```python
from build123d import *

# Parameters (mm, degrees)
F0_W          = 571.5
F0_H          = 19.05
F1_DEPTH      = 88.9
F2_W          = 88.9
F2_H          = 19.05
F3_DEPTH      = 6.35
F4_W          = 88.9
F4_H          = 19.05
F5_DEPTH      = 6.35
F5_DEPTH_BACK = 25.4


with BuildPart() as f1:
    # F0 (on Front) → F1 (new body, symmetric)
    with BuildSketch(Plane.XZ):
        with Locations((285.75, 9.525)):
            Rectangle(F0_W, F0_H)
    extrude(amount=F1_DEPTH, both=True)

    # F2 (on face) → F3 (join)
    with BuildSketch(Plane.YZ.offset(571.5)):
        with Locations((44.45, 9.525)):
            Rectangle(F2_W, F2_H)
    extrude(amount=F3_DEPTH)

    # F4 (on face) → F5 (join, two sides)
    with BuildSketch(Plane(origin=(0, 0, 0), x_dir=(0, -1, 0), z_dir=(-1, 0, 0))) as f5_sk:
        with Locations((-44.45, 9.525)):
            Rectangle(F4_W, F4_H)
    extrude(amount=F5_DEPTH)
    extrude(f5_sk.sketch, amount=-F5_DEPTH_BACK)


solid = f1.part
```
The listing builds one solid part. Answer for the finished solid, in the listing's coordinates (mm). A direction names the side the tool comes from. Coordinates: 2 decimals unless noted, no trailing zeros. Loops run counter-clockwise (first coordinate to the right, second up) from the corner with the lowest first, then second, coordinate; pieces in that order, holes last. Notation, with made-up numbers: (32.25, 61.25) -> (85.25, 61.25) arc R18 ccw to (85.25, 95.25) -> close; hole circle Ø2 at (5.25, 61). An arc over 180 degrees is marked (long way). Use one line per item in the form item = value. Start each with the question number.
Item 1: The part is cut by section A-A on y = -72.5. Determine the outline of the cut face in (x, z).
Item 2: Consider L1, parallel to X at y = -68.5, z = 13.25. Determine where the line is inside the solid, lowest interval first. Write a range as [from, to].
Item 3: Flat-ended cylindrical pins translate along their axes: pin 1 Ø9.5 at (y, z) = (-29.5, 9) entering from -X; pin 2 Ø5.5 at (y, z) = (-36, 5) entering from +X; pin 3 Ø5 at (x, z) = (-3.5, 12) entering from -Y. Find the tip coordinate at first contact, or state that the pin passes through.
Item 4: A tool of negligible diameter and unlimited length cuts with its end or side. For faces 1 (the face through (290, 1, 0)), 2 (the face through (571.5, -45, 9)), 3 (the face through (0, -45, 9)), from which of +Z, -Z, +X, -X, +Y, -Y can it reach the whole face along a straight path? Write none if from no direction.
Answer key:
q1.outline = (0, 0) -> (571.5, 0) -> (571.5, 19.05) -> (0, 19.05) -> close
q2.L1 = [0, 571.5]
q3.pin_1 = 0
q3.pin_2 = 571.5
q3.pin_3 = 0
q4.face_1 = -Z, +X, -X, +Y, -Y
q4.face_2 = +Z, -Z, +X, -Y
q4.face_3 = +Z, -Z, -X, -Y
